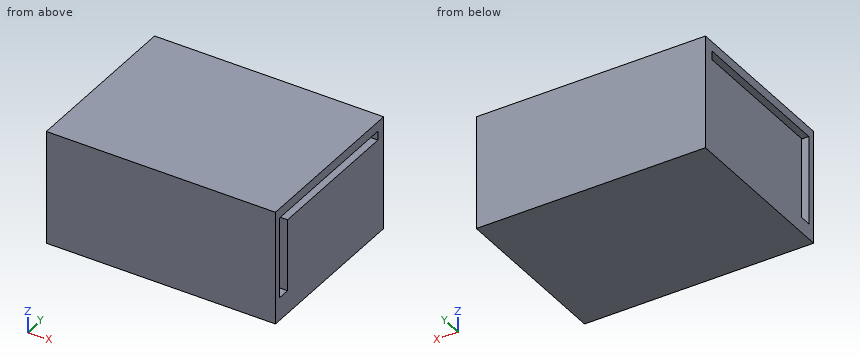
```python
from build123d import *

# Parameters (mm, degrees)
F0_W     = 151.777678
F0_H     = 151.339829
F1_DEPTH = 100.584
F2_W     = 151.339829
F2_H     = 100.584
F3_DEPTH = 25.4
F4_W     = 151.339829
F4_H     = 100.584
F5_DEPTH = 25.4


with BuildPart() as f1:
    # F0 (on Top) → F1 (new body)
    with BuildSketch(Plane.XY):
        with Locations((-0.823509, 1.426369)):
            Rectangle(F0_W, F0_H)
    extrude(amount=F1_DEPTH)

    # F2 (on face) → F3 (join)
    with BuildSketch(Plane.YZ.offset(75.06533)):
        with Locations((1.426369, 50.292)):
            Rectangle(F2_W, F2_H)
        Polygon((-68.466783, 20.36312), (-68.466783, 84.190369), (-68.466783, 92.207313), (-57.366394, 92.207313), (69.054723, 92.207313), (69.054723, 84.190369), (-57.366394, 84.190369), (-57.366394, 20.36312), align=None, mode=Mode.SUBTRACT)
    extrude(amount=F3_DEPTH)

    # F4 (on face) → F5 (join)
    with BuildSketch(Plane(origin=(-76.712348, 0, 0), x_dir=(0, -1, 0), z_dir=(-1, 0, 0))):
        with Locations((-1.426369, 50.292)):
            Rectangle(F4_W, F4_H)
        Polygon((56.951661, 92.207313), (67.435369, 92.207313), (67.435369, 84.498711), (67.435369, 13.579548), (56.951661, 13.579548), (56.951661, 84.498711), (-67.927733, 84.498711), (-67.927733, 92.207313), align=None, mode=Mode.SUBTRACT)
    extrude(amount=F5_DEPTH)


solid = f1.part
```
Can you work these out from the model? Positions are in its coordinate system, mm. Coordinates: 2 decimals unless noted, no trailing zeros. Order: outer loops, then holes, each group sorted by start corner. A loop starts at its lowest first (then second) coordinate and runs counter-clockwise, first axis right, second up. Notation, with made-up numbers: (-4.75, -2) -> (3.25, -2) arc R22 ccw to (3.25, 10) -> close; hole circle Ø2 at (82.25, -2). An arc over 180 degrees is marked (long way). Write each question's results on one line, items separated by ' | '.
Item 1: I want a section at A-A, the plane x = 79.5. Write out the boundary of the cut face in (y, z).
Results are:
outline: (-74.24, 0) -> (77.1, 0) -> (77.1, 100.58) -> (-74.24, 100.58) -> close; hole (-68.47, 20.36) -> (-57.37, 20.36) -> (-57.37, 84.19) -> (69.05, 84.19) -> (69.05, 92.21) -> (-68.47, 92.21) -> close
Item 2: I want a section at B-B, the plane z = 57. Write out the boundary of the cut face in (x, y).
Results are:
outline: (-102.11, -74.24) -> (100.47, -74.24) -> (100.47, -68.47) -> (75.07, -68.47) -> (75.07, -57.37) -> (100.47, -57.37) -> (100.47, 77.1) -> (-102.11, 77.1) -> (-102.11, -56.95) -> (-76.71, -56.95) -> (-76.71, -67.44) -> (-102.11, -67.44) -> close
Item 3: If I drill on line 1 along Z through (x, y) = (-85, -51.5); line 2 along Y through (x, z) = (87, 27); line 3 along X through (y, z) = (29, 91), over which ranges is the centre line in solid material (lowest first)?
Results are:
line 1: 0 to 84.5, 92.21 to 100.58 | line 2: -74.24 to -68.47, -57.37 to 77.1 | line 3: -76.71 to 75.07
Item 4: I want a section at C-C, the plane y = -14.5. Write out the boundary of the cut face in (x, z).
Results are:
outline: (-102.11, 0) -> (100.47, 0) -> (100.47, 84.19) -> (75.07, 84.19) -> (75.07, 92.21) -> (100.47, 92.21) -> (100.47, 100.58) -> (-102.11, 100.58) -> (-102.11, 92.21) -> (-76.71, 92.21) -> (-76.71, 84.5) -> (-102.11, 84.5) -> close
